Autodesk Inventor part; units mm, degrees
ref_plane "YZ Plane" through (0, 0, 0) normal (1, 0, 0) x (0, 1, 0)
ref_plane "XZ Plane" through (0, 0, 0) normal (0, 1, 0) x (-1, 0, 0)
ref_plane "XY Plane" through (0, 0, 0) normal (0, 0, 1) x (1, 0, 0)
sketch "Sketch1" plane through (0, 0, 0) normal (0, 0, 1) x (1, 0, 0)
  line L0 (0, 0) -> (45, 0) construction
  line L1 (45, 0) -> (45, 20) construction
  line L2 (45, 20) -> (0, 20) construction
  line L3 (0, 20) -> (0, 0) construction
  line L4 (0, 0) -> (9, 0) construction
  line L5 (9, 0) -> (9, 10) construction
  line L6 (45, 0) -> (36, 0) construction
  line L7 (36, 0) -> (36, 10) construction
  circle A0 centre (36, 10) radius 8
  circle A1 centre (9, 10) radius 8
  line L8 (45, 0) -> (46, 0) construction
  line L9 (46, 0) -> (46, -1) construction
  line L10 (0, 20) -> (-1, 20) construction
  line L11 (-1, 20) -> (-1, 21) construction
  line L12 (-1, 21) -> (46, 21)
  line L13 (46, 21) -> (46, -1)
  line L14 (46, -1) -> (-1, -1)
  line L15 (-1, -1) -> (-1, 21)
  line L16 (45, 0) -> (0, 0)
  line L17 (0, 0) -> (0, 20)
  line L18 (0, 20) -> (45, 20)
  line L19 (45, 20) -> (45, 0)
  dimension "d2" = 45
  dimension "d3" = 20
  dimension "d4" = 9
  dimension "d5" = 10
  dimension "d6" = 9
  dimension "d7" = 10
  dimension "d8" = 16
  dimension "d9" = 16
  dimension "d10" = 1
  dimension "d11" = 1
  dimension "d12" = 1
  dimension "d13" = 1
extrude "Extrusion1" add sketch "Sketch1" along normal blind 9.169 contours L12 L13 L14 L15 | L16 L17 L18 L19
sketch "Sketch2" plane through (0, 0, 0) normal (0, 0, -1) x (-1, 0, 0)
  line L0 (0, 0) -> (-45, 0)
  line L1 (-45, 0) -> (-45, 20)
  line L2 (-45, 20) -> (0, 20)
  line L3 (0, 20) -> (0, 0)
  dimension "d14" = 45
  dimension "d15" = 20
extrude "Extrusion2" cut sketch "Sketch2" against normal blind 3.169
sketch "Sketch3" plane through (-1, -1, 0) normal (0, -1, 0) x (1, 0, 0)
  line L0 (47, 0) -> (47, 9.169) construction
  line L1 (47, 4.5845) -> (0, 4.5845) construction
  line L2 (0, 0) -> (0, 9.169) construction
  line L3 (47, 0) -> (0, 0) construction
  line L4 (23.5, 0) -> (23.5, 9.169) construction
  line L5 (0, 9.169) -> (47, 9.169) construction
  line L6 (23.5, 4.5845) -> (23.5, 2.3345) construction
  line L7 (23.5, 2.3345) -> (21.25, 2.3345) construction
  line L8 (21.25, 2.3345) -> (13.15, 2.3345) construction
  line L9 (13.15, 2.3345) -> (8.65, 2.3345) construction
  line L10 (8.65, 2.3345) -> (0.55, 2.3345) construction
  line L11 (0.55, 2.3345) -> (-3.95, 2.3345) construction
  line L12 (-3.95, 2.3345) -> (-12.05, 2.3345) construction
  line L13 (23.5, 2.3345) -> (25.75, 2.3345) construction
  line L14 (25.75, 2.3345) -> (33.85, 2.3345) construction
  line L15 (33.85, 2.3345) -> (38.35, 2.3345) construction
  line L16 (38.35, 2.3345) -> (46.45, 2.3345) construction
  line L17 (46.45, 2.3345) -> (50.95, 2.3345) construction
  line L18 (50.95, 2.3345) -> (59.05, 2.3345) construction
  line L19 (21.25, 2.3345) -> (25.75, 2.3345)
  line L20 (25.75, 2.3345) -> (25.75, 6.8345)
  line L21 (25.75, 6.8345) -> (21.25, 6.8345)
  line L22 (21.25, 6.8345) -> (21.25, 2.3345)
  line L23 (8.65, 2.3345) -> (13.15, 2.3345)
  line L24 (13.15, 2.3345) -> (13.15, 6.8345)
  line L25 (13.15, 6.8345) -> (8.65, 6.8345)
  line L26 (8.65, 6.8345) -> (8.65, 2.3345)
  line L27 (38.35, 2.3345) -> (33.85, 2.3345)
  line L28 (33.85, 2.3345) -> (33.85, 6.8345)
  line L29 (33.85, 6.8345) -> (38.35, 6.8345)
  line L30 (38.35, 6.8345) -> (38.35, 2.3345)
  line L31 (13.15, 2.3345) -> (14.15, 2.3345) construction
  line L32 (14.15, 2.3345) -> (14.15, 1.3345) construction
  line L33 (8.65, 6.8345) -> (8.65, 7.8345) construction
  line L34 (8.65, 7.8345) -> (7.65, 7.8345) construction
  line L35 (7.65, 7.8345) -> (14.15, 7.8345)
  line L36 (14.15, 7.8345) -> (14.15, 1.3345)
  line L37 (14.15, 1.3345) -> (7.65, 1.3345)
  line L38 (7.65, 1.3345) -> (7.65, 7.8345)
  line L39 (25.75, 2.3345) -> (26.75, 2.3345) construction
  line L40 (26.75, 2.3345) -> (26.75, 1.3345) construction
  line L41 (21.25, 6.8345) -> (21.25, 7.8345) construction
  line L42 (21.25, 7.8345) -> (20.25, 7.8345) construction
  line L43 (33.85, 6.8345) -> (32.85, 6.8345) construction
  line L44 (32.85, 6.8345) -> (32.85, 7.8345) construction
  line L45 (38.35, 2.3345) -> (39.35, 2.3345) construction
  line L46 (39.35, 2.3345) -> (39.35, 1.3345) construction
  line L47 (26.75, 1.3345) -> (20.25, 1.3345)
  line L48 (20.25, 1.3345) -> (20.25, 7.8345)
  line L49 (20.25, 7.8345) -> (26.75, 7.8345)
  line L50 (26.75, 7.8345) -> (26.75, 1.3345)
  line L51 (39.35, 1.3345) -> (32.85, 1.3345)
  line L52 (32.85, 1.3345) -> (32.85, 7.8345)
  line L53 (32.85, 7.8345) -> (39.35, 7.8345)
  line L54 (39.35, 7.8345) -> (39.35, 1.3345)
  point P0 (1, 0)
  dimension "d18" = 2.25
  dimension "d19" = 2.25
  dimension "d20" = 8.1
  dimension "d21" = 4.5
  dimension "d22" = 8.1
  dimension "d23" = 4.5
  dimension "d24" = 8.1
  dimension "d25" = 2.25
  dimension "d26" = 8.1
  dimension "d27" = 4.5
  dimension "d28" = 8.1
  dimension "d29" = 4.5
  dimension "d30" = 8.1
  dimension "d31" = 4.5
  dimension "d32" = 4.5
  dimension "d33" = 4.5
  dimension "d34" = 4.5
  dimension "d35" = 4.5
  dimension "d36" = 4.5
  dimension "d37" = 1
  dimension "d38" = 1
  dimension "d39" = 1
  dimension "d40" = 1
  dimension "d41" = 1
  dimension "d42" = 1
  dimension "d43" = 1
  dimension "d44" = 1
  dimension "d45" = 1
  dimension "d46" = 1
  dimension "d47" = 1
  dimension "d48" = 1
extrude "Extrusion3" add sketch "Sketch3" along normal blind 7
equation "\"d2\" = wsonar"
equation "\"d3\" = hsonar"
equation "\"d10\" = thickness"
equation "\"d11\" = thickness"
equation "\"d12\" = thickness"
equation "\"d13\" = thickness"
equation "\"d14\" = wsonar"
equation "\"d15\" = hsonar"
equation "\"d18\" = 0.5 * box"
equation "\"d19\" = 0.5 * box"
equation "\"d20\" = gap"
equation "\"d21\" = box"
equation "\"d22\" = gap"
equation "\"d23\" = box"
equation "\"d24\" = gap"
equation "\"d25\" = 0.5 * box"
equation "\"d26\" = gap"
equation "\"d27\" = box"
equation "\"d28\" = gap"
equation "\"d29\" = box"
equation "\"d30\" = gap"
equation "\"d31\" = box"
equation "\"d32\" = box"
equation "\"d33\" = box"
equation "\"d34\" = box"
equation "\"d35\" = box"
equation "\"d36\" = box"
equation "\"d37\" = thickness"
equation "\"d38\" = thickness"
equation "\"d39\" = thickness"
equation "\"d40\" = thickness"
equation "\"d41\" = thickness"
equation "\"d42\" = thickness"
equation "\"d43\" = thickness"
equation "\"d44\" = thickness"
equation "\"d45\" = thickness"
equation "\"d46\" = thickness"
equation "\"d47\" = thickness"
equation "\"d48\" = thickness"
equation "\"wsonar\" = 45"
equation "\"hsonar\" = 20"
equation "\"thickness\" = 1"
equation "\"gap\" = 8.1"
equation "\"box\" = 4.5"
properties part number "Sonar"
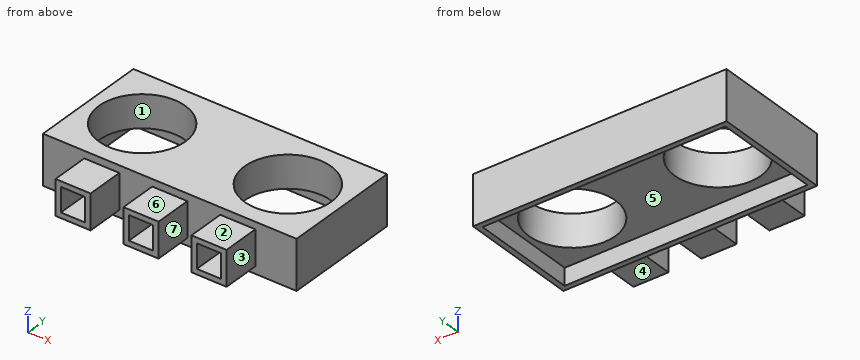
Verification items for the finished model (mm, model axes). Face numbers are marked on the shaded views. A direction names the side the tool comes from. Give positions to 0.01 mm unless a question says otherwise; leave off trailing zeros. Order: outer loops, then holes, each group sorted by start corner. A loop starts at its lowest first (then second) coordinate and runs counter-clockwise, first axis right, second up. Notation, with made-up numbers: M 34.5,-19.75 L 49.5,-19.75 A17 ccw 49.5,-4.75 Z; hole C -36.75,4.25 d9. An arc over 180 degrees is marked long. Use one line per item in the form item = value. Start each with the question number.
Q1. Section check A-A (x = 9). Enter the section's corners in (y, z).
Q2. Access from +Z, -Z, +X, -X, +Y, -Y to the whole of each face (thin tool, end or side, straight path). Record for the marked faces 4, 5, 6 and 7.
Q3. Section check B-B (y = -1.5). Enter the section's corners in (x, z), then the cut area to 3 significant figures.
Q4. Go/stop test with flat-tipped pins: pin 1 Ø1.3 at (y, z) = (-3.5, 5) entering from -X; pin 2 Ø3.5 at (y, z) = (-4, 5.5) entering from +X; pin 3 Ø9.5 at (x, y) = (9, 10) entering from +Z; pin 4 Ø2 at (x, y) = (9.5, -5) entering from +Z. Record where each tip stops, or that it passes through.
Q5. Section check D-D (y = 10). Enter the section's corners in (x, z), then the cut area to 3 significant figures.
Q6. Section check C-C (z = 4.5). Count the separate pieces of the cut face and the enclosed holes in it, then the cut area to 3 significant figures.
Q7. Mould release check, pull along X, two halves, no side actions. Record for the marked faces 1, 2 and 3: +X half, -X half, draft (parallel to the pull), parting line (faces both ways), or undercut.
Q8. Scan lines: line 1 along X through (y, z) = (10, 7.3); line 2 along Y through (x, z) = (34, 0.75); line 3 along Y through (x, z) = (36, 6.65). Record each from-to range of solid material in increasing order. Write a range as [from, to].
Evaluation:
q1.outline = M -8,1.33 L -1,1.33 L -1,0 L 0,0 L 0,3.17 L 2,3.17 L 2,9.17 L -1,9.17 L -1,7.83 L -8,7.83 L -8,6.83 L -1,6.83 L -1,2.33 L -8,2.33 Z; M 18,3.17 L 20,3.17 L 20,0 L 21,0 L 21,9.17 L 18,9.17 Z
q2.face_4 = -Z, +X, -X, -Y
q2.face_5 = -Z
q2.face_6 = +Z, +X, -X, -Y
q2.face_7 = +Z, -Z, -Y
q3.outline = M 6.65,1.33 L 13.15,1.33 L 13.15,7.83 L 6.65,7.83 Z; M 19.25,1.33 L 25.75,1.33 L 25.75,7.83 L 19.25,7.83 Z; M 31.85,1.33 L 38.35,1.33 L 38.35,7.83 L 31.85,7.83 Z; hole M 7.65,2.33 L 12.15,2.33 L 12.15,6.83 L 7.65,6.83 Z; hole M 20.25,2.33 L 24.75,2.33 L 24.75,6.83 L 20.25,6.83 Z; hole M 32.85,2.33 L 37.35,2.33 L 37.35,6.83 L 32.85,6.83 Z
q3.area = 66.0 mm2
q4.pin_1 = 6.65
q4.pin_2 = 38.35
q4.pin_3 = through
q4.pin_4 = 7.83
q5.outline = M -1,0 L 0,0 L 0,3.17 L 1,3.17 L 1,9.17 L -1,9.17 Z; M 17,3.17 L 28,3.17 L 28,9.17 L 17,9.17 Z; M 44,3.17 L 45,3.17 L 45,0 L 46,0 L 46,9.17 L 44,9.17 Z
q5.area = 96.3 mm2
q6.separate_pieces = 1
q6.enclosed_holes = 2
q6.area = 674 mm2
q7.face_1 = undercut
q7.face_2 = draft
q7.face_3 = +X half
q8.line_1 = [-1, 1], [17, 28], [44, 46]
q8.line_2 = [-1, 0], [20, 21]
q8.line_3 = [-1, 2], [18, 21]
